Build history of the part. All positions in model axes, mm. Face numbers are marked on the shaded views. A direction names the side the tool comes from. Round coordinates to 2 decimals unless told otherwise and drop trailing zeros. Loops run counter-clockwise (first coordinate to the right, second up) from the corner with the lowest first, then second, coordinate; pieces in that order, holes last. Notation, with made-up numbers: (14, 82) - (45, 82) arc R18 cw to (45, 89) - close; hole circle Ø5 at (17, -38). An arc over 180 degrees is marked (long way). Use a Markdown table: item, result.
from build123d import *

# Parameters (mm, degrees)
SZKIC1_R                    = 11
SZKIC1_R_2                  = 4
DODANIE_WYCI_GNI_CIE1_DEPTH = 3.5
SZKIC2_R                    = 9.184724544
SZKIC2_R_2                  = 5.450254851
WYTNIJ_WYCI_GNI_CIE1_DEPTH  = 0.2
ZAOKR_GLENIE1_R             = 0.5


with BuildPart() as part:
    # Szkic1 → Dodanie-wyciągnięcie1 (new body, symmetric)
    with BuildSketch(Plane.XY):
        Circle(SZKIC1_R)
        Circle(SZKIC1_R_2, mode=Mode.SUBTRACT)
    extrude(amount=DODANIE_WYCI_GNI_CIE1_DEPTH, both=True)

    # Szkic2 → Wytnij-wyciągnięcie1 (cut)
    with BuildSketch(Plane.XY.offset(3.5)):
        Circle(SZKIC2_R)
        Circle(SZKIC2_R_2, mode=Mode.SUBTRACT)
    wytnij_wyci_gni_cie1 = extrude(amount=-WYTNIJ_WYCI_GNI_CIE1_DEPTH, mode=Mode.SUBTRACT)

    # Lustro1: Wytnij-wyciągnięcie1 across plane
    add(wytnij_wyci_gni_cie1.mirror(Plane.XY), mode=Mode.SUBTRACT)

    # Zaokrąglenie1
    zaokr_glenie1_edges = [part.edges().sort_by_distance(p)[0] for p in [
        (-11, 0, -3.5),
        (-11, 0, 3.5),
        (-4, 0, -3.5),
        (-4, 0, 3.5),
    ]]
    fillet(zaokr_glenie1_edges, radius=ZAOKR_GLENIE1_R)


solid = part.part
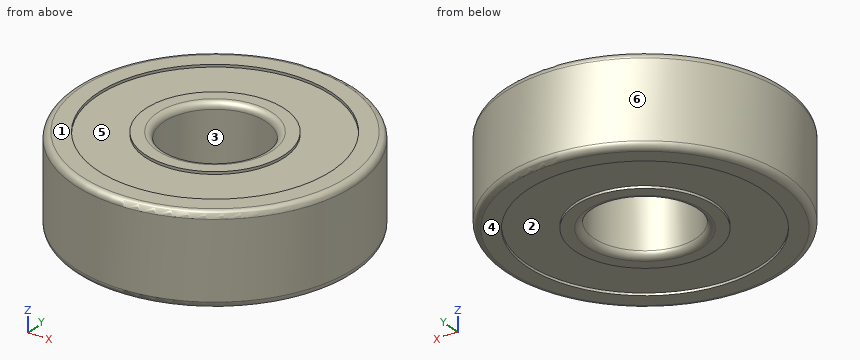
Q1. Drop flat-ended pins along their axis: pin 1 (2 mm diameter, centred on y = 2, z = 2, fed in from -X); pin 2 (4 mm diameter, centred on x = 4.5, z = -2.5, fed in from +Y). Give the stop position or say it passes through.
Results found:
| item | result |
|---|---|
| pin 1 | stops at x = -10.95 |
| pin 2 | stops at y = 10.71 |
Q2. Probe line 1 (Y direction, x = 0, z = -3.35); line 2 (Y direction, x = 0, z = 3.4); line 3 (Y direction, x = 0, z = 1.5). List the from-to ranges inside material, lowest first.
Results found:
| item | result |
|---|---|
| line 1 | y = -10.86 to -9.18, -5.45 to -4.14, 4.14 to 5.45, 9.18 to 10.86 |
| line 2 | y = -10.8 to -9.18, -5.45 to -4.2, 4.2 to 5.45, 9.18 to 10.8 |
| line 3 | y = -11 to -4, 4 to 11 |
Q3. Which spindle directions (+Z, -Z, +X, -X, +Y, -Y) get a long thin tool onto all of the face, cutting with end or side? Do the marked faces 1 and 2. Say none if no direction does.
Results found:
| item | result |
|---|---|
| face 1 | +Z, +X, -X, +Y, -Y |
| face 2 | -Z |
Q4. Cut at C-C, the plane z = 1.5. List the corners of the cut face in (x, y).
Results found:
| item | result |
|---|---|
| outline | circle Ø22 at (0, 0); hole circle Ø8 at (0, 0) |
Q5. Pull direction X, two halves, no side cores. Call the marked faces 3, 4, 5 and 6: pulls with the +X half, pulls with the -X half, needs draft (parallel to the pull), parting line crosses it, or undercut.
Results found:
| item | result |
|---|---|
| face 3 | undercut |
| face 4 | needs draft |
| face 5 | undercut |
| face 6 | parting line crosses it |
